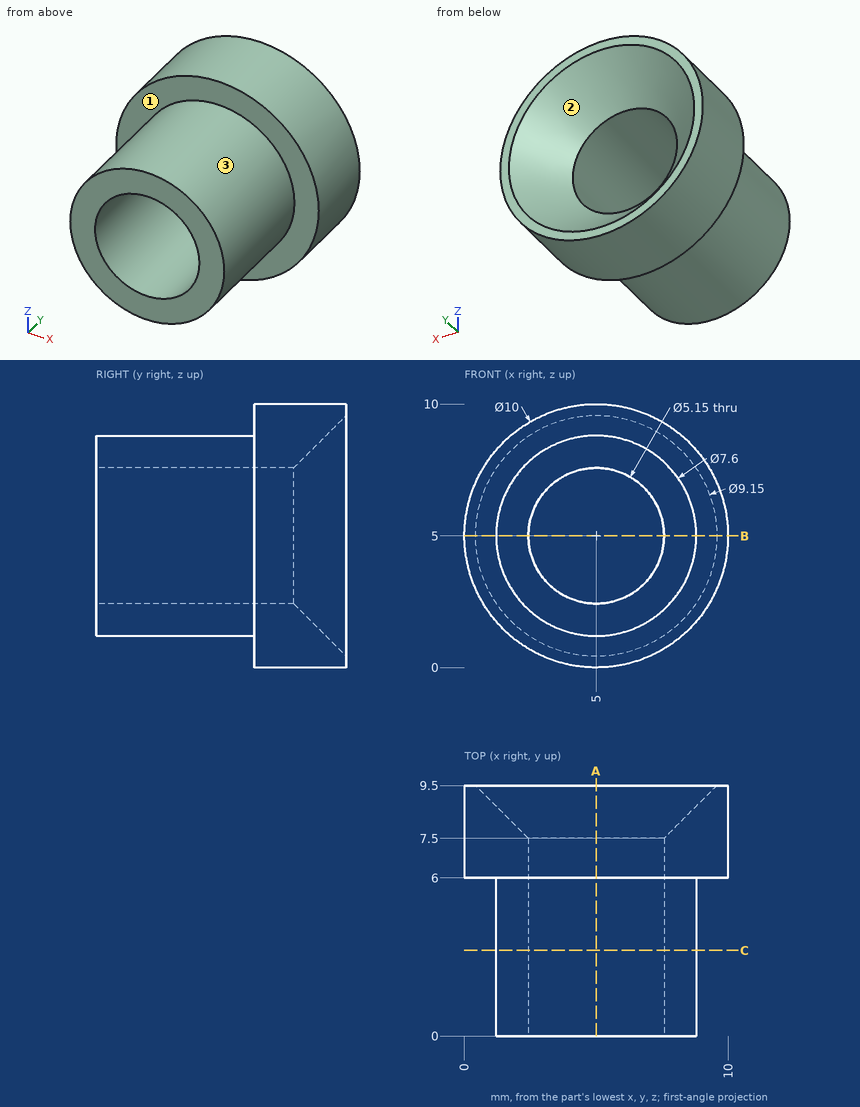
The drawing under review shows one solid part. Ordinate dimensions are in mm from its lowest x, y, z. Coordinates: 2 decimals unless noted, no trailing zeros. Order: outer loops, then holes, each group sorted by start corner. A loop starts at its lowest first (then second) coordinate and runs counter-clockwise, first axis right, second up. Notation, with made-up numbers: (57.5, 52) - (78.5, 52) arc R21 ccw to (78.5, 75) - close; hole circle Ø11 at (74, 10). An arc over 180 degrees is marked (long way). Put each result on its own line as item: value.
1) Take a section at C-C, the plane y = 3.25. Give the boundary of the cut face in (x, z) (3 decimals), and give its area (3 significant figures).
Response values:
outline: circle Ø7.6 at (5, 5); hole circle Ø5.15 at (5, 5)
area: 24.5 mm²
2) Take a section at B-B, the plane z = 5. Give the boundary of the cut face in (x, y) (3 decimals), and give its area (3 significant figures).
Response values:
outline: (0, 6) - (1.2, 6) - (1.2, 0) - (2.425, 0) - (2.425, 7.5) - (0.425, 9.5) - (0, 9.5) - close; (7.575, 0) - (8.8, 0) - (8.8, 6) - (10, 6) - (10, 9.5) - (9.575, 9.5) - (7.575, 7.5) - close
area: 27.7 mm²
3) Wall thickness on L1, parallel to Z at x = 5, y = 5.5 (3 decimals); L2, parallel to X at y = 9, z = 7; L3, parallel to X at y = 1, z = 7: over which ranges is each line inside the solid? List them lowest first. Write a range as from..to.
Response values:
L1: z = 1.2..2.425, 7.575..8.8
L2: x = 0.42..1.45, 8.55..9.58
L3: x = 1.77..3.38, 6.62..8.23
4) Take a section at A-A, the plane x = 5. Give the boundary of the cut face in (y, z) (3 decimals).
Response values:
outline: (0, 1.2) - (6, 1.2) - (6, 0) - (9.5, 0) - (9.5, 0.425) - (7.5, 2.425) - (0, 2.425) - close; (0, 7.575) - (7.5, 7.575) - (9.5, 9.575) - (9.5, 10) - (6, 10) - (6, 8.8) - (0, 8.8) - close
5) Insertion check: P1, Ø3, axis at x = 3, y = 1.5, coming from the +Z side; P2, Ø1.5, axis at y = 3, z = 1, coming from the -X side; P3, Ø2, axis at x = 7, y = 1.5, coming from the -Z side. Each pin has a flat end and moves straight along its axis. Give the tip position at first contact, or say it passes through.
Response values:
P1: stops at z = 8.77
P2: stops at x = 3.03
P3: stops at z = 1.33
6) The part is to be moulded in two halves that separate along X. For the marked faces 1, 2 and 3, say which applies: released by +X, released by -X, zero draft, split by the parting line, or undercut.
Response values:
face 1: zero draft
face 2: undercut
face 3: split by the parting line
